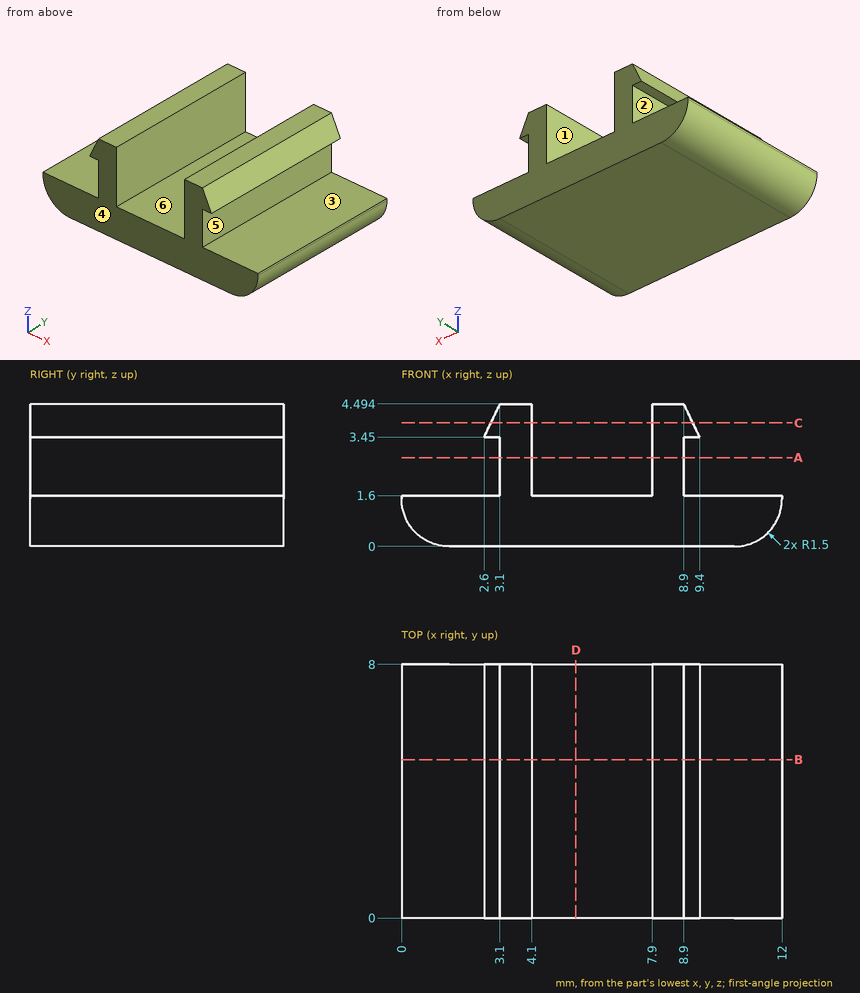
The drawing under review shows one solid part. Ordinate dimensions are in mm from its lowest x, y, z. A direction names the side the tool comes from. Round coordinates to 2 decimals unless told otherwise and drop trailing zeros. Write each loop counter-clockwise with the first axis right and the second up, starting at its lowest first coordinate (ties: lowest second). Pieces come first, ordered by that corner, then holes. Notation, with made-up numbers: (-12.5, 36) - (2.5, 36) arc R16 ccw to (2.5, 45) - close; hole circle Ø6 at (-1.5, 83). An arc over 180 degrees is marked (long way). Put each result on its own line as item: value.
Q1. We need section B-B (y = 5). Give the boundary of the cut face in (x, z).
Solved:
outline: (0, 1.5) arc R1.5 ccw to (1.5, 0) - (10.5, 0) arc R1.5 ccw to (12, 1.5) - (12, 1.6) - (8.9, 1.6) - (8.9, 3.45) - (9.4, 3.45) - (8.9, 4.49) - (7.9, 4.49) - (7.9, 1.6) - (4.1, 1.6) - (4.1, 4.49) - (3.1, 4.49) - (2.6, 3.45) - (3.1, 3.45) - (3.1, 1.6) - (0, 1.6) - close
Q2. Mouldability with a two-part tool opening along Z and no side actions: class the marked faces 4, 5 and 6 as released by +Z, released by -Z, zero draft, split by the parting line, or undercut.
Solved:
face 4: zero draft
face 5: undercut
face 6: released by +Z
Q3. We need section C-C (z = 3.9). Give the boundary of the cut face in (x, y) (1 decimal).
Solved:
outline: (2.8, 0) - (4.1, 0) - (4.1, 8) - (2.8, 8) - close; (7.9, 0) - (9.2, 0) - (9.2, 8) - (7.9, 8) - close
Q4. Machinability: for the marked faces 1, 2 and 3, which of the approach directions +Z, -Z, +X, -X, +Y, -Y give a long, thin tool a straight path to every point of the face, cutting with its end or side? Answer none if there is none.
Solved:
face 1: +Z, +Y, -Y
face 2: -X, +Y, -Y
face 3: +X, +Y, -Y
Q5. Wall thickness on probe 1 along Z at (x, y) = (5, 3.75); probe 2 along X at (y, z) = (6.5, 3.75) (1 decimal); probe 3 along X at (y, z) = (5.75, 0.8) (1 decimal): over which ranges is each line inside the solid? List them lowest first.
Solved:
probe 1: z = 0 to 1.6
probe 2: x = 2.7 to 4.1, 7.9 to 9.3
probe 3: x = 0.2 to 11.8
Q6. Insertion check: pin 1 Ø2 at (y, z) = (3, 3) entering from +X; pin 2 Ø1 at (y, z) = (1, 3.5) entering from -X; pin 3 Ø0.9 at (y, z) = (5.5, 2.5) entering from +X. Each pin has a flat end and moves straight along its axis. Give the tip position at first contact, or say it passes through.
Solved:
pin 1: stops at x = 9.4
pin 2: stops at x = 2.6
pin 3: stops at x = 8.9
Q7. We need section D-D (x = 5.5). Give the boundary of the cut face in (y, z).
Solved:
outline: (0, 0) - (8, 0) - (8, 1.6) - (0, 1.6) - close
Q8. We need section A-A (z = 2.8). Give the boundary of the cut face in (x, y), and give its area (3 significant figures).
Solved:
outline: (3.1, 0) - (4.1, 0) - (4.1, 8) - (3.1, 8) - close; (7.9, 0) - (8.9, 0) - (8.9, 8) - (7.9, 8) - close
area: 16.0 mm2
